Design review of the part shown in the three views and the two pictorial views. Dimensions are in mm from the part's minimum x, y and z. A direction names the side the tool comes from. Coordinates: 2 decimals unless noted, no trailing zeros. Write each loop counter-clockwise with the first axis right and the second up, starting at its lowest first coordinate (ties: lowest second). Pieces come first, ordered by that corner, then holes.
Q1. Take a section at B-B, the plane z = 7. Write out the cut boundary in (x, y), plus the area to 3 significant figures.
Q2. For pin 1 Ø5.5 at (x, z) = (7, 7) entering from +Y; pin 2 Ø2 at (y, z) = (3, 4) entering from -X; pin 3 Ø1 at (y, z) = (0.5, 11.5) entering from -X, all flat-tipped, find the tip position at first contact; note any pin that passes through.
Q3. Take a section at A-A, the plane x = 7. Write out the cut boundary in (y, z).
Q4. Take a section at D-D, the plane z = 10.75. Write out the cut boundary in (x, y), plus the area to 3 significant figures.
Q5. The part is to be moulded in two halves that separate along X. For the marked faces 1, 2 and 3, say which applies: released by +X, released by -X, zero draft, split by the parting line, or undercut.
Q6. Take a section at C-C, the plane y = 3.15. Write out the cut boundary in (x, z).
Q7. For the marked faces 4, 5 and 6, list the 3-axis set-ups (+Z, -Z, +X, -X, +Y, -Y) from which the entire face can be reached by the end or side of a thin tool; tool diameter is ignored.
Q8. For L1, parallel to X at y = 3.9, z = 7; L2, parallel to X at y = 1.3, z = 7; L3, parallel to Y at x = 6.25, z = 5.75, list the stretches that pass through material, from the lowest coordinate up.
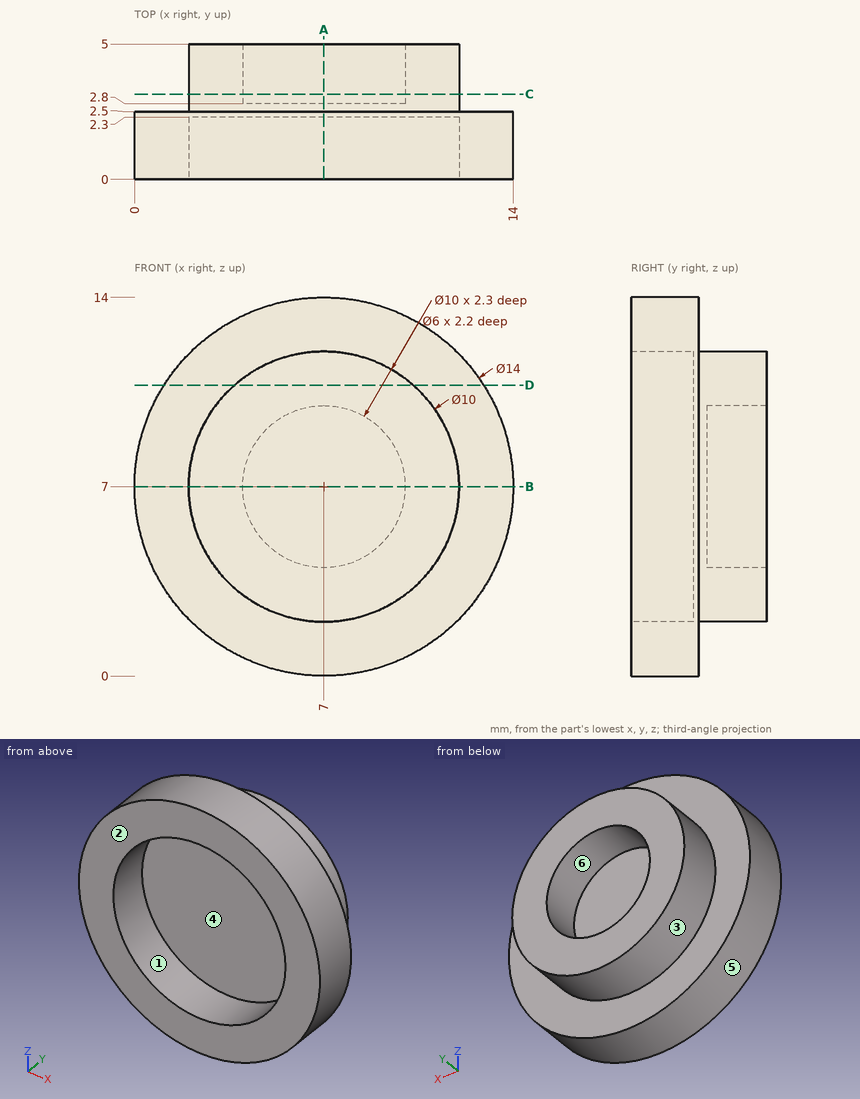
Responses:
1. outline: (0, 0) - (2, 0) - (2, 2.3) - (12, 2.3) - (12, 0) - (14, 0) - (14, 2.5) - (12, 2.5) - (12, 5) - (10, 5) - (10, 2.8) - (4, 2.8) - (4, 5) - (2, 5) - (2, 2.5) - (0, 2.5) - close
1. area: 23.8 mm2
2. pin 1: stops at y = 2.8
2. pin 2: stops at x = 0.33
2. pin 3: stops at x = 1.26
3. outline: (0, 0) - (2.5, 0) - (2.5, 2) - (5, 2) - (5, 4) - (2.8, 4) - (2.8, 10) - (5, 10) - (5, 12) - (2.5, 12) - (2.5, 14) - (0, 14) - (0, 12) - (2.3, 12) - (2.3, 2) - (0, 2) - close
4. outline: (1.09, 0) - (3.69, 0) - (3.69, 2.3) - (10.31, 2.3) - (10.31, 0) - (12.91, 0) - (12.91, 2.5) - (10.31, 2.5) - (10.31, 5) - (3.69, 5) - (3.69, 2.5) - (1.09, 2.5) - close
4. area: 30.9 mm2
5. face 1: undercut
5. face 2: zero draft
5. face 3: split by the parting line
6. outline: circle Ø10 at (7, 7); hole circle Ø6 at (7, 7)
7. face 4: -Y
7. face 5: +Y, -Y
7. face 6: +Y
8. L1: x = 2 to 4, 10 to 12
8. L2: x = 0 to 2, 12 to 14
8. L3: y = 2.3 to 2.8
